from build123d import *

# Parameters (mm, degrees)
F0_W        = 2
F0_H        = 5
F1_DEPTH    = 6
F2_T        = 2.5
F2_T3_DEPTH = 11


# Not quite as in the source:
# - a shell that OpenCascade refuses in one call is made with other operations: the cavity is built on its own and cut out


with BuildPart() as f1:
    # F0 (on Top) → F1 (new body)
    with BuildSketch(Plane.XY):
        Polygon((30, 0), (0, 0), (0, -10), (14, -10), (14, -5), (16, -5), (16, -10), (30, -10), align=None)
        with Locations((15, -7.5)):
            Rectangle(F0_W, F0_H)
        with Locations((15, -12.5)):
            Rectangle(F0_W, F0_H)
    extrude(amount=F1_DEPTH)

    # F2: shell of thickness 2.5, made by hand


with BuildPart() as f2_core1:
    # F2_t2: copy of F1
    add(f1.part)

    # the walls: a layer under each face that stays
    f2_faces = [f2_core1.faces().sort_by_distance(p)[0] for p in [
        (15, 0, 3),
        (0, -5, 3),
        (7, -10, 3),
        (14, -12.5, 3),
        (15, -15, 3),
        (16, -12.5, 3),
        (23, -10, 3),
        (30, -5, 3),
        (15, -7.5, 0),
    ]]
    thicken(f2_faces, amount=-F2_T, mode=Mode.SUBTRACT)

    # F2_s4 → F2_t3 (cut)
    with BuildSketch(Plane.XY.offset(-2.5)):
        Polygon((13.975, -10.025), (14, -7.5), (16.5, -7.5), (16.5, -10), align=None)
        Polygon((16.025, -10.025), (13.5, -10), (13.5, -7.5), (16, -7.5), align=None)
    extrude(amount=F2_T3_DEPTH, mode=Mode.SUBTRACT)


with BuildPart() as f1_1:
    add(f1.part)

    # what is left inside the walls is the cavity
    f2_cavity = [f2_core1.part.solids().sort_by_distance(p)[0] for p in [
        (15, -5.833333, 5.975),
    ]]
    add(f2_cavity, mode=Mode.SUBTRACT)


solid = f1_1.part
Could you check a few things on this model? Use its own coordinates, in mm. A direction names the side the tool comes from. Coordinates: 2 decimals unless noted, no trailing zeros. Write each loop counter-clockwise with the first axis right and the second up, starting at its lowest first coordinate (ties: lowest second). Pieces come first, ordered by that corner, then holes. Notation, with made-up numbers: (23, -16.75) - (82, -16.75) arc R33 ccw to (82, 13.25) - close; hole circle Ø1 at (43.5, 9). An arc over 180 degrees is marked (long way). Write item = value, one per line.
1) Suppose I cut it at B-B on y = -6.5. Please give me the cut outline in (x, z).
Result set:
outline = (0, 0) - (30, 0) - (30, 6) - (27.5, 6) - (27.5, 2.5) - (2.5, 2.5) - (2.5, 6) - (0, 6) - close
2) Suppose I cut it at A-A on z = 3.65. Please give me the cut outline in (x, y).
Result set:
outline = (0, -10) - (14, -10) - (14, -15) - (16, -15) - (16, -10) - (30, -10) - (30, 0) - (0, 0) - close; hole (2.5, -7.5) - (27.5, -7.5) - (27.5, -2.5) - (2.5, -2.5) - close
3) For faces 1 (the flat face through (7, -10, 3)), 2 (the flat face through (15, -7.5, 4)), 3 (the flat face through (23, -10, 3)), which set-ups out of +Z, -Z, +X, -X, +Y, -Y let a thin tool reach every point of the face, with its end or its side?
Result set:
face_1 = +Z, -Z, -X, -Y
face_2 = +Z
face_3 = +Z, -Z, +X, -Y
4) Suppose I cut it at D-D on x = 2. Please give me the cut outline in (y, z), plus the area to 3 significant figures.
Result set:
outline = (-10, 0) - (0, 0) - (0, 6) - (-10, 6) - close
area = 60.0 mm2
5) Will this pin go through, and if not, where does the flat tip stop? pin 1 Ø1 at (x, z) = (20, 5) entering from -Y.
Result set:
pin_1 = -10
6) Suppose I cut it at C-C on x = 11.75. Please give me the cut outline in (y, z).
Result set:
outline = (-10, 0) - (0, 0) - (0, 6) - (-2.5, 6) - (-2.5, 2.5) - (-7.5, 2.5) - (-7.5, 6) - (-10, 6) - close
7) We'd pull the mould along X, two halves only. Please class faces 4 (the flat face through (2.5, -5, 4)), 5 (the flat face through (16, -13, 3)), 6 (the flat face through (0, -5, 3)), 7 (the flat face through (27.5, -5, 4)): +X half, -X half, draft (parallel to the pull), parting line (faces both ways), or undercut.
Result set:
face_4 = undercut
face_5 = +X half
face_6 = -X half
face_7 = undercut
8) Please list where these lines run through material, in increasing order: line 1 (Y direction, x = 13, z = 2.9); line 2 (X direction, y = -7, z = 4.2); line 3 (Y direction, x = 4, z = 0.4). Write a range as [from, to].
Result set:
line_1 = [-10, -7.5], [-2.5, 0]
line_2 = [0, 2.5], [27.5, 30]
line_3 = [-10, 0]
